Can you work these out from the model? Positions are in its coordinate system, mm. Face numbers are marked on the shaded views. A direction names the side the tool comes from. Round coordinates to 2 decimals unless told otherwise and drop trailing zeros. Loops run counter-clockwise (first coordinate to the right, second up) from the corner with the lowest first, then second, coordinate; pieces in that order, holes last.
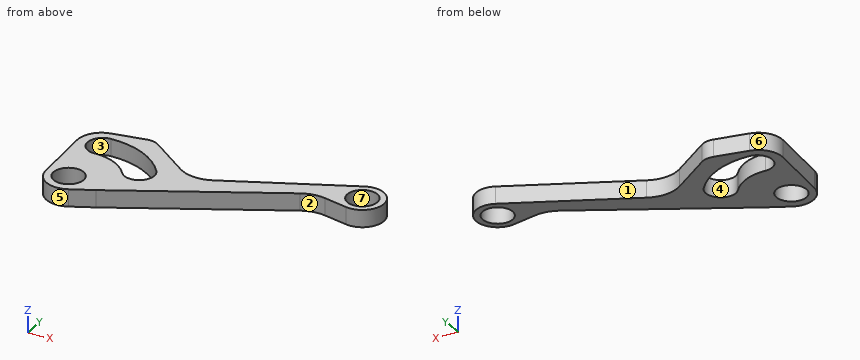
from build123d import *

# Parameters (mm, degrees)
SKETCH2_R           = 1.75
BOSS_EXTRUDE1_DEPTH = 2
SCALE1_SCALE        = 2


with BuildPart() as part:
    # Sketch2 → Boss-Extrude1 (new body)
    with BuildSketch(Plane.XY):
        with BuildLine():
            Line((-2.959686812, 7.094235734), (-2.589510897, -0.112410482))
            ThreePointArc((-2.589510897, -0.112410482), (-1.247895547, -2.342588234), (1.351636108, -2.469315214))
            Line((1.351636108, -2.469315214), (3.894134078, -1.267559521))
            Line((3.894134078, -1.267559521), (22.318004544, 8.181471599))
            ThreePointArc((22.318004544, 8.181471599), (23.631672458, 8.589402593), (25.00585725, 8.528187863))
            Line((25.00585725, 8.528187863), (27.810968992, 7.908802431))
            ThreePointArc((27.810968992, 7.908802431), (30.836871293, 10.605873355), (27.325176398, 12.630293092))
            Line((27.325176398, 12.630293092), (13.285071523, 6.320301234))
            ThreePointArc((13.285071523, 6.320301234), (11.187238244, 5.995090505), (9.218440829, 6.78913284))
            Line((9.218440829, 6.78913284), (4.711624461, 10.229038009))
            ThreePointArc((4.711624461, 10.229038009), (3.977045573, 10.581042261), (3.163031294, 10.61094026))
            Line((3.163031294, 10.61094026), (-0.662699736, 9.960674362))
            ThreePointArc((-0.662699736, 9.960674362), (-2.356294969, 8.964265917), (-2.959686812, 7.094235734))
        make_face()
        Circle(SKETCH2_R, mode=Mode.SUBTRACT)
        with Locations((28.35, 10.35)):
            Circle(SKETCH2_R, mode=Mode.SUBTRACT)
        with BuildLine():
            ThreePointArc((-0.062114538, 8.972511771), (-1.799958067, 7.210439165), (-0.037885462, 5.472595636))
            ThreePointArc((-0.037885462, 5.472595636), (2.468926518, 4.884172412), (4.429179601, 3.21451495))
            ThreePointArc((4.429179601, 3.21451495), (6.873384478, 2.826104706), (7.261794722, 5.270309583))
            ThreePointArc((7.261794722, 5.270309583), (4.047891296, 8.007771334), (-0.062114538, 8.972511771))
        make_face(mode=Mode.SUBTRACT)
    extrude(amount=BOSS_EXTRUDE1_DEPTH)


with BuildPart() as part_1:
    # Scale1: scaled about (9.442389577, 5.344617661, 1)
    add(part.part.scale(SCALE1_SCALE).moved(Location((-9.442389577, -5.344617661, -1))))


solid = part_1.part
(1) If we section it at D-D, the plane x = 39: List the corners of the cut face in (y, z) for me.
Worked answers:
outline: (11.9, -1) - (17.13, -1) - (17.13, 3) - (11.9, 3) - close
(2) If we mould it in two halves opening along X, with no side actions, what happens to the marked faces 4, 5, 6 and 7? For each: released by +X, released by -X, zero draft, split by the parting line, or undercut.
Worked answers:
face 4: undercut
face 5: split by the parting line
face 6: released by -X
face 7: undercut
(3) If we section it at A-A, the plane y = 3: List the corners of the cut face in (x, z) for me, then the cut area to 3 significant figures.
Worked answers:
outline: (-15.06, -1) - (-2.36, -1) - (-2.36, 3) - (-15.06, 3) - close; (5.75, -1) - (19.56, -1) - (19.56, 3) - (5.75, 3) - close
area: 106 mm2
(4) If we section it at C-C, the plane y = -6.5: List the corners of the cut face in (x, z) for me, then the cut area to 3 significant figures.
Worked answers:
outline: (-14.49, -1) - (-12.75, -1) - (-12.75, 3) - (-14.49, 3) - close; (-6.14, -1) - (1.04, -1) - (1.04, 3) - (-6.14, 3) - close
area: 35.7 mm2
(5) If we section it at B-B, the plane z = -0.2: List the corners of the cut face in (x, y) for me.
Worked answers:
outline: (-15.36, 8.84) - (-14.62, -5.57) arc R5.53 ccw to (-6.74, -10.28) - (-1.65, -7.88) - (35.19, 11.02) arc R8 cw to (40.57, 11.71) - (46.18, 10.47) arc R5 ccw (long way) to (45.21, 19.92) - (17.13, 7.3) arc R8 cw to (8.99, 8.23) - (-0.02, 15.11) arc R4 ccw to (-3.12, 15.88) - (-10.77, 14.58) arc R5.53 ccw to start; hole circle Ø7 at (-9.44, -5.34); hole (-9.57, 12.6) arc R3.5 ccw to (-9.52, 5.6) arc R10.95 cw to (-0.58, 1.08) arc R3.5 ccw to (5.08, 5.2) arc R17.95 ccw to start; hole circle Ø7 at (47.26, 15.36)
(6) If I drill on line 1 (Y direction, x = 47, z = 0.35); line 2 (Y direction, x = -9, z = 0.85); line 3 (X direction, y = 16.5, z = 1), over which ranges is the centre line in solid material (lowest first)?
Worked answers:
line 1: y = 10.36 to 11.86, 18.85 to 20.35
line 2: y = -10.81 to -8.82, -1.87 to 5.59, 12.6 to 14.88
line 3: x = 37.61 to 43.95, 50.57 to 52.12
(7) For the marked faces 1, 2 and 3, which set-ups out of +Z, -Z, +X, -X, +Y, -Y let a thin tool reach every point of the face, with its end or its side?
Worked answers:
face 1: +Z, -Z, +Y
face 2: +Z, -Z, -Y
face 3: +Z, -Z
(8) Will these pins go through, and if not, where does the flat tip stop? P1, Ø8, axis at x = 0.5, y = 4, coming from the +Z side; P2, Ø2, axis at x = 31.5, z = 0, coming from the -Y side; P3, Ø6.5, axis at x = 47.26, y = 15.36, coming from the +Z side; P4, Ø1, axis at x = 7.5, z = 0.5, coming from the -Y side.
Worked answers:
P1: stops at z = 3
P2: stops at y = 8.61
P3: passes through
P4: stops at y = -3.44
